Can you work these out from the model? Positions are in its coordinate system, mm. Face numbers are marked on the shaded views. Round coordinates to 2 decimals unless told otherwise and drop trailing zeros. Loops run counter-clockwise (first coordinate to the right, second up) from the corner with the lowest first, then second, coordinate; pieces in that order, holes last. Notation, with made-up numbers: M 38.25,69 L 60.25,69 A14 ccw 60.25,87 Z; hole C 48,15 d7. An arc over 180 degrees is marked long. Return JSON: item names as keys, results as strings.
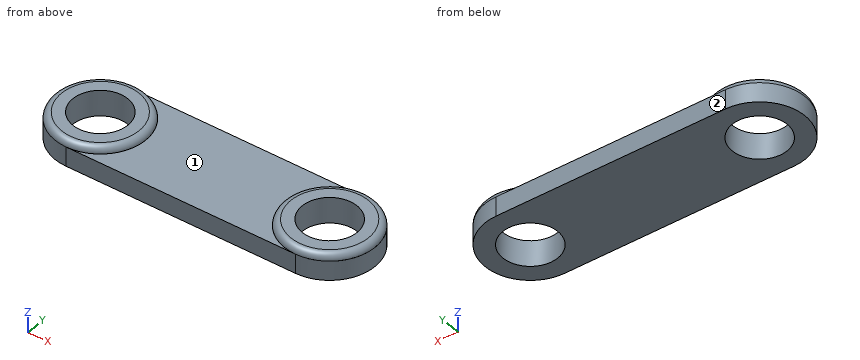
```python
from build123d import *
from build123d.topology import SkipClean

# Parameters (mm, degrees)
SKETCH1_R           = 4.25
SKETCH1_W           = 20
SKETCH1_H           = 5
BOSS_EXTRUDE1_DEPTH = 3
SKETCH2_R           = 7
SKETCH2_R_2         = 4.25
BOSS_EXTRUDE2_DEPTH = 1
FILLET1_R           = 1
CUT_EXTRUDE1_DEPTH  = 48.11952886


with BuildPart() as part:
    # Sketch1 → Boss-Extrude1 (new body)
    with BuildSketch(Plane.XY):
        with BuildLine():
            Line((9, -33.5), (-26, -33.5))
            ThreePointArc((-26, -33.5), (-33, -26.5), (-26, -19.5))
            Line((-26, -19.5), (-20, -19.5))
            ThreePointArc((-20, -19.5), (-16.464466094, -18.035533906), (-15, -14.5))
            Line((-15, -14.5), (-15, 28.5))
            ThreePointArc((-15, 28.5), (-13.535533906, 32.035533906), (-10, 33.5))
            Line((-10, 33.5), (10, 33.5))
            ThreePointArc((10, 33.5), (13.535533906, 32.035533906), (15, 28.5))
            Line((15, 28.5), (15, -22.894448725))
            ThreePointArc((15, -22.894448725), (15.092571663, -29.946820352), (9, -33.5))
        make_face()
        with Locations((9, -26.5)):
            Circle(SKETCH1_R, mode=Mode.SUBTRACT)
        with Locations((-26, -26.5)):
            Circle(SKETCH1_R, mode=Mode.SUBTRACT)
        with Locations((0, 26)):
            Rectangle(SKETCH1_W, SKETCH1_H, mode=Mode.SUBTRACT)
    extrude(amount=BOSS_EXTRUDE1_DEPTH)

    # Sketch2 → Boss-Extrude2 (add)
    # profile 1 of 2: a face of its own
    with BuildSketch(Plane.XY.offset(3)):
        with Locations(Location((-26, -26.5, 0), (0, 0, 270))):
            Circle(SKETCH2_R)
        with Locations((-26, -26.5)):
            Circle(SKETCH2_R_2, mode=Mode.SUBTRACT)
    # profile 2 of 2: a face of its own
    with BuildSketch(Plane.XY.offset(3)):
        with Locations(Location((9, -26.5, 0), (0, 0, 270))):
            Circle(SKETCH2_R)
        with Locations((9, -26.5)):
            Circle(SKETCH2_R_2, mode=Mode.SUBTRACT)
    extrude(amount=BOSS_EXTRUDE2_DEPTH)

    # Fillet1
    fillet1_edges = [part.edges().sort_by_distance(p)[0] for p in [
        (-26, -19.5, 4),
        (9, -19.5, 4),
    ]]
    fillet(fillet1_edges, radius=FILLET1_R - 0.0001)  # a hair under: the kernel refuses the full size

    # Sketch3 → Cut-Extrude1 (cut, through all)
    with SkipClean():  # the faces are left unmerged after this step: merging them gives an invalid solid
        with BuildSketch(Plane.XY.offset(3)):
            with BuildLine():
                Line((-20, -19.5), (9, -19.5))
                ThreePointArc((9, -19.5), (12.446820352, -20.407428337), (15, -22.894448725))
                Line((15, -22.894448725), (15, 33.5))
                Line((15, 33.5), (-20, 33.5))
                Line((-20, 33.5), (-20, -19.5))
            make_face()
        extrude(amount=-CUT_EXTRUDE1_DEPTH, mode=Mode.SUBTRACT)


solid = part.part
```
Q1. Suppose I cut it at B-B, the plane z = 0.7. Please give me the cut outline in (x, y), plus the area to 3 significant figures.
Results:
{"outline": "M -26,-33.5 L 9,-33.5 A7 ccw 9,-19.5 L -26,-19.5 A7 ccw Z; hole C -26,-26.5 d8.5; hole C 9,-26.5 d8.5", "area": "530 mm2"}
Q2. Thinking about a two-plate mould opening in X: for the marked faces 1 and 2, which applies, pulls with the +X half, pulls with the -X half, needs draft (parallel to the pull), parting line crosses it, or undercut?
Results:
{"face 1": "undercut", "face 2": "needs draft"}
Q3. Suppose I cut it at A-A, the plane y = -26.5. State how many separate pieces and enclosed holes the cut face has, plus the area to 3 significant figures.
Results:
{"separate pieces": "3", "enclosed holes": "0", "area": "106 mm2"}
Q4. Suppose I cut it at C-C, the plane x = -3. Please give me the cut outline in (y, z), plus the area to 3 significant figures.
Results:
{"outline": "M -33.5,0 L -19.5,0 L -19.5,3 L -33.5,3 Z", "area": "42.0 mm2"}
Q5. If I drill on line 1 along X through (y, z) = (-29.5, 0.65); line 2 along Y through (x, z) = (-26, 0.95); line 3 along Z through (x, y) = (-18.5, -31.25), over which ranges is the centre line in solid material (lowest first)?
Results:
{"line 1": "x = -32.32 to -29.01, -22.99 to 5.99, 12.01 to 15.32", "line 2": "y = -33.5 to -30.75, -22.25 to -19.5", "line 3": "z = 0 to 3"}
Q6. I'm going to push flat-ended pins straight in: pin 1 Ø2 at (x, y) = (3.5, -31) entering from +Z; pin 2 Ø1 at (y, z) = (-23.5, 2) entering from -X; pin 3 Ø5 at (x, y) = (-26, -26.5) entering from +Z; pin 4 Ø2 at (y, z) = (-25, 3) entering from -X. Where does each tip first touch, or does it pass through?
Results:
{"pin 1": "stops at z = 3.99", "pin 2": "stops at x = -32.54", "pin 3": "passes through", "pin 4": "stops at x = -32.98"}
